Check sheet for the modelled part. Datum: model origin and axes. Units: mm. Give positions to 0.01 mm unless a question says otherwise; leave off trailing zeros.
from build123d import *

# Parameters (mm, degrees)
SKETCH2_W           = 100
SKETCH2_H           = 160
SKETCH2_R           = 1.3
BOSS_EXTRUDE1_DEPTH = 2
SKETCH3_W           = 14
SKETCH3_H           = 20
CUT_EXTRUDE1_DEPTH  = 2
FILLET1_R           = 1.5


with BuildPart() as part:
    # Sketch2 → Boss-Extrude1 (new body)
    with BuildSketch(Plane(origin=(0, 0, 0), x_dir=(1, 0, 0), z_dir=(0, 1, 0))):
        Rectangle(SKETCH2_W, SKETCH2_H)
        with Locations(Location((22.422835534, 63.736544033, 0), (0, 0, 270))):
            Circle(SKETCH2_R, mode=Mode.SUBTRACT)
        with Locations(Location((22.422835534, 71.514718626, 0), (0, 0, 270))):
            Circle(SKETCH2_R, mode=Mode.SUBTRACT)
        with Locations(Location((28.079689783, 77.171572875, 0), (0, 0, 270))):
            Circle(SKETCH2_R, mode=Mode.SUBTRACT)
        with Locations(Location((46, 13.5, 0), (0, 0, 270))):
            Circle(SKETCH2_R, mode=Mode.SUBTRACT)
        with Locations(Location((38, 13.5, 0), (0, 0, 270))):
            Circle(SKETCH2_R, mode=Mode.SUBTRACT)
        with Locations(Location((32.5, 8, 0), (0, 0, 270))):
            Circle(SKETCH2_R, mode=Mode.SUBTRACT)
        with Locations(Location((32.5, -8, 0), (0, 0, 90))):
            Circle(SKETCH2_R, mode=Mode.SUBTRACT)
        with Locations(Location((38, -13.5, 0), (0, 0, 90))):
            Circle(SKETCH2_R, mode=Mode.SUBTRACT)
        with Locations(Location((46, -13.5, 0), (0, 0, 90))):
            Circle(SKETCH2_R, mode=Mode.SUBTRACT)
        with Locations(Location((47.171572875, 58.079689783, 0), (0, 0, 90))):
            Circle(SKETCH2_R, mode=Mode.SUBTRACT)
        with Locations(Location((41.514718626, 52.422835534, 0), (0, 0, 90))):
            Circle(SKETCH2_R, mode=Mode.SUBTRACT)
        with Locations(Location((33.736544033, 52.422835534, 0), (0, 0, 90))):
            Circle(SKETCH2_R, mode=Mode.SUBTRACT)
        with Locations(Location((47.171572875, -58.079689783, 0), (0, 0, 270))):
            Circle(SKETCH2_R, mode=Mode.SUBTRACT)
        with Locations(Location((41.514718626, -52.422835534, 0), (0, 0, 270))):
            Circle(SKETCH2_R, mode=Mode.SUBTRACT)
        with Locations(Location((33.736544033, -52.422835534, 0), (0, 0, 270))):
            Circle(SKETCH2_R, mode=Mode.SUBTRACT)
        with Locations(Location((28.079689783, -77.171572875, 0), (0, 0, 90))):
            Circle(SKETCH2_R, mode=Mode.SUBTRACT)
        with Locations(Location((22.422835534, -71.514718626, 0), (0, 0, 90))):
            Circle(SKETCH2_R, mode=Mode.SUBTRACT)
        with Locations(Location((22.422835534, -63.736544033, 0), (0, 0, 90))):
            Circle(SKETCH2_R, mode=Mode.SUBTRACT)
        with Locations(Location((-28.079689783, 77.171572875, 0), (0, 0, 90))):
            Circle(SKETCH2_R, mode=Mode.SUBTRACT)
        with Locations(Location((-22.422835534, 71.514718626, 0), (0, 0, 90))):
            Circle(SKETCH2_R, mode=Mode.SUBTRACT)
        with Locations(Location((-22.422835534, 63.736544033, 0), (0, 0, 90))):
            Circle(SKETCH2_R, mode=Mode.SUBTRACT)
        with Locations(Location((-47.171572875, 58.079689783, 0), (0, 0, 270))):
            Circle(SKETCH2_R, mode=Mode.SUBTRACT)
        with Locations(Location((-41.514718626, 52.422835534, 0), (0, 0, 270))):
            Circle(SKETCH2_R, mode=Mode.SUBTRACT)
        with Locations(Location((-33.736544033, 52.422835534, 0), (0, 0, 270))):
            Circle(SKETCH2_R, mode=Mode.SUBTRACT)
        with Locations(Location((-47.171572875, -58.079689783, 0), (0, 0, 90))):
            Circle(SKETCH2_R, mode=Mode.SUBTRACT)
        with Locations(Location((-41.514718626, -52.422835534, 0), (0, 0, 90))):
            Circle(SKETCH2_R, mode=Mode.SUBTRACT)
        with Locations(Location((-33.736544033, -52.422835534, 0), (0, 0, 90))):
            Circle(SKETCH2_R, mode=Mode.SUBTRACT)
        with Locations(Location((-22.422835534, -63.736544033, 0), (0, 0, 270))):
            Circle(SKETCH2_R, mode=Mode.SUBTRACT)
        with Locations(Location((-22.422835534, -71.514718626, 0), (0, 0, 270))):
            Circle(SKETCH2_R, mode=Mode.SUBTRACT)
        with Locations(Location((-28.079689783, -77.171572875, 0), (0, 0, 270))):
            Circle(SKETCH2_R, mode=Mode.SUBTRACT)
        with Locations(Location((-32.5, -8, 0), (0, 0, 270))):
            Circle(SKETCH2_R, mode=Mode.SUBTRACT)
        with Locations(Location((-38, -13.5, 0), (0, 0, 270))):
            Circle(SKETCH2_R, mode=Mode.SUBTRACT)
        with Locations(Location((-46, -13.5, 0), (0, 0, 270))):
            Circle(SKETCH2_R, mode=Mode.SUBTRACT)
        with Locations(Location((-46, 13.5, 0), (0, 0, 90))):
            Circle(SKETCH2_R, mode=Mode.SUBTRACT)
        with Locations(Location((-38, 13.5, 0), (0, 0, 90))):
            Circle(SKETCH2_R, mode=Mode.SUBTRACT)
        with Locations(Location((-32.5, 8, 0), (0, 0, 90))):
            Circle(SKETCH2_R, mode=Mode.SUBTRACT)
    extrude(amount=BOSS_EXTRUDE1_DEPTH)

    # Sketch3 → Cut-Extrude1 (cut)
    with BuildSketch(Plane(origin=(0, 2, 0), x_dir=(1, 0, 0), z_dir=(0, 1, 0))):
        with Locations((43, 0)):
            Rectangle(SKETCH3_W, SKETCH3_H)
        Polygon((35.857864376, 80), (23.129942315, 67.272077939), (37.272077939, 53.129942315), (50, 65.857864376), (50, 80), align=None)
        Polygon((50, -65.857864376), (50, -80), (35.857864376, -80), (23.129942315, -67.272077939), (37.272077939, -53.129942315), align=None)
        Polygon((-50, 65.857864376), (-50, 80), (-35.857864376, 80), (-23.129942315, 67.272077939), (-37.272077939, 53.129942315), align=None)
        with Locations((-43, 0)):
            Rectangle(SKETCH3_W, SKETCH3_H)
        Polygon((-37.272077939, -53.129942315), (-50, -65.857864376), (-50, -80), (-35.857864376, -80), (-23.129942315, -67.272077939), align=None)
    extrude(amount=-CUT_EXTRUDE1_DEPTH, mode=Mode.SUBTRACT)

    # Fillet1
    fillet1_edges = [part.edges().sort_by_distance(p)[0] for p in [
        (35.857864376, 1, -80),
        (50, 1, -65.857864376),
        (50, 1, 65.857864376),
        (35.857864376, 1, 80),
        (-50, 1, -65.857864376),
        (-35.857864376, 1, -80),
        (-50, 1, 10),
        (-50, 1, -10),
        (-35.857864376, 1, 80),
        (-50, 1, 65.857864376),
        (50, 1, -10),
        (50, 1, 10),
    ]]
    fillet(fillet1_edges, radius=FILLET1_R)


solid = part.part
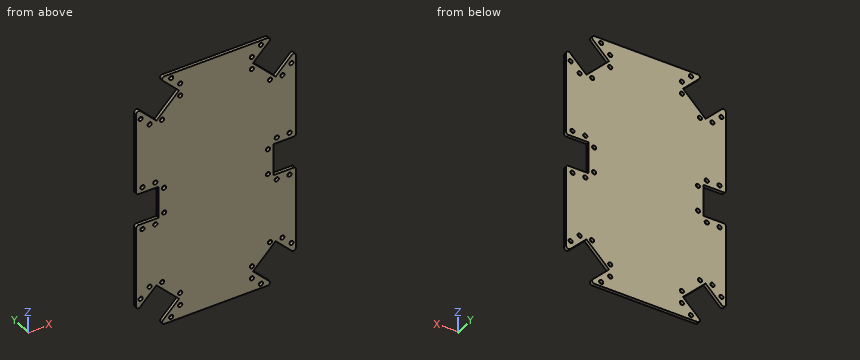
1) Section check A-A, the plane y = 0.7. State how many separate pieces and enclosed holes the cut face has, then the cut area to 3 significant figures.
Recorded:
separate pieces: 1
enclosed holes: 36
area: 13,400 mm2
2) Material ranges on L1, parallel to X at y = 0.7, z = -13.5; L2, parallel to Z at x = 28.5, y = 1.65; L3, parallel to X at y = 0.45, z = -63, recorded low to high.
Recorded:
L1: x = -50 to -47.3, -44.7 to -39.3, -36.7 to 36.7, 39.3 to 44.7, 47.3 to 50
L2: z = -80 to -78.4, -75.94 to -72.64, -61.9 to 61.9, 72.64 to 75.94, 78.4 to 80
L3: x = -49.79 to -47.14, -27.4 to -23.49, -21.35 to 21.35, 23.49 to 27.4, 47.14 to 49.79
3) Depth check by flat-ended pin: pin 1 Ø2.5 at (x, z) = (-33.74, -52.42) entering from -Y; pin 2 Ø1 at (y, z) = (1, 7) entering from -X. Enter the tip coordinate at first touch or a pass-through.
Recorded:
pin 1: passes through
pin 2: stops at x = -36
